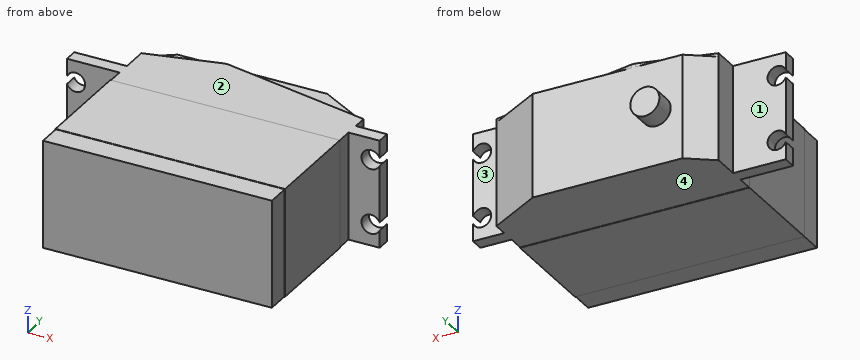
from build123d import *

# Parameters (mm, degrees)
SKETCH2_W            = 66
SKETCH2_H            = 31
BOSS_EXTRUDE1_DEPTH  = 44.6
SKETCH4_W            = 31
SKETCH4_H            = 3.9
BOSS_EXTRUDE2_DEPTH  = 9
SKETCH6_R            = 2.75
CUT_EXTRUDE3_DEPTH   = 64.193433203
BOSS_EXTRUDE4_DEPTH  = 3.9
SKETCH8_W            = 66
SKETCH8_H            = 31
BOSS_EXTRUDE5_DEPTH  = 12.96
CUT_EXTRUDE7_DEPTH   = 82.21610038
CUT_EXTRUDE8_DEPTH   = 82.21610038
CUT_EXTRUDE9_DEPTH   = 1
SKETCH12_R           = 4.19
BOSS_EXTRUDE6_DEPTH  = 6
SKETCH13_W           = 66
SKETCH13_H           = 29.265979079
BOSS_EXTRUDE7_DEPTH  = 0.1
SKETCH14_W           = 31.1
SKETCH14_H           = 29.164669929
BOSS_EXTRUDE8_DEPTH  = 0.1
SKETCH15_W           = 66.1
SKETCH15_H           = 29.164669929
BOSS_EXTRUDE9_DEPTH  = 0.1
SKETCH16_W           = 31.2
SKETCH16_H           = 29.265979079
BOSS_EXTRUDE10_DEPTH = 0.1


with BuildPart() as part:
    # Sketch2 → Boss-Extrude1 (new body)
    with BuildSketch(Plane(origin=(0, 0, 0), x_dir=(1, 0, 0), z_dir=(0, 1, 0))):
        Rectangle(SKETCH2_W, SKETCH2_H)
    extrude(amount=BOSS_EXTRUDE1_DEPTH)

    # Sketch4 → Boss-Extrude2 (add)
    with BuildSketch(Plane(origin=(33, 0, 0), x_dir=(0, 0, -1), z_dir=(1, 0, 0))):
        with Locations((0, 42.65)):
            Rectangle(SKETCH4_W, SKETCH4_H)
    extrude(amount=BOSS_EXTRUDE2_DEPTH)

    # Sketch6 → Cut-Extrude3 (cut, through all)
    with BuildSketch(Plane(origin=(0, 44.6, 0), x_dir=(1, 0, 0), z_dir=(0, 1, 0))):
        with Locations((39.5, -9.35)):
            Circle(SKETCH6_R)
        with Locations((39.5, 9.35)):
            Circle(SKETCH6_R)
    extrude(amount=-CUT_EXTRUDE3_DEPTH, mode=Mode.SUBTRACT)

    # Sketch7 → Boss-Extrude4 (add)
    with BuildSketch(Plane(origin=(0, 44.6, 0), x_dir=(1, 0, 0), z_dir=(0, 1, 0))):
        with BuildLine():
            Line((-33, 15.5), (-48.186111703, 15.5))
            Line((-48.186111703, 15.5), (-48.186111703, 10.495643924))
            ThreePointArc((-48.186111703, 10.495643924), (-42.936111703, 9.35), (-48.186111703, 8.204356076))
            Line((-48.186111703, 8.204356076), (-48.186111703, -8.204356076))
            ThreePointArc((-48.186111703, -8.204356076), (-42.936111703, -9.35), (-48.186111703, -10.495643924))
            Line((-48.186111703, -10.495643924), (-48.186111703, -15.5))
            Line((-48.186111703, -15.5), (-33, -15.5))
            Line((-33, -15.5), (-33, 15.5))
        make_face()
    extrude(amount=-BOSS_EXTRUDE4_DEPTH)

    # Sketch8 → Boss-Extrude5 (add)
    with BuildSketch(Plane(origin=(0, 44.6, 0), x_dir=(1, 0, 0), z_dir=(0, 1, 0))):
        Rectangle(SKETCH8_W, SKETCH8_H)
    extrude(amount=BOSS_EXTRUDE5_DEPTH)

    # Sketch9 → Cut-Extrude7 (cut, through all)
    with BuildSketch(Plane.XY.offset(15.5)):
        Polygon((-25.417976584, 57.56), (-33, 52.251010049), (-33, 57.56), align=None)
    extrude(amount=-CUT_EXTRUDE7_DEPTH, mode=Mode.SUBTRACT)

    # Sketch10 → Cut-Extrude8 (cut, through all)
    with BuildSketch(Plane.XY.offset(15.5)):
        Polygon((17.751890933, 57.56), (33, 48.756500125), (33, 57.56), align=None)
    extrude(amount=-CUT_EXTRUDE8_DEPTH, mode=Mode.SUBTRACT)

    # Sketch11 → Cut-Extrude9 (cut)
    with BuildSketch(Plane.XY.offset(15.5)):
        Polygon((-33, 52.251010049), (-11.889467425, 57.56), (-25.417976584, 57.56), align=None)
        Polygon((33, 48.756500125), (-10.755426907, 57.56), (17.751890933, 57.56), align=None)
    extrude(amount=-CUT_EXTRUDE9_DEPTH, mode=Mode.SUBTRACT)

    # Sketch12 → Boss-Extrude6 (add)
    with BuildSketch(Plane(origin=(0, 57.56, 0), x_dir=(1, 0, 0), z_dir=(0, 1, 0))):
        with Locations(Location((-17.839262747, 0, 0), (0, 0, 270))):
            Circle(SKETCH12_R)
    extrude(amount=BOSS_EXTRUDE6_DEPTH)

    # Sketch13 → Boss-Extrude7 (add)
    with BuildSketch(Plane(origin=(0, 0, -15.5), x_dir=(-1, 0, 0), z_dir=(0, 0, -1))):
        with Locations((0, 21.440452746)):
            Rectangle(SKETCH13_W, SKETCH13_H)
    extrude(amount=BOSS_EXTRUDE7_DEPTH)

    # Sketch14 → Boss-Extrude8 (add)
    with BuildSketch(Plane.ZY.offset(33)):
        with Locations((-0.05, 21.389798171)):
            Rectangle(SKETCH14_W, SKETCH14_H)
    extrude(amount=BOSS_EXTRUDE8_DEPTH)

    # Sketch15 → Boss-Extrude9 (add)
    with BuildSketch(Plane.XY.offset(15.5)):
        with Locations((-0.05, 21.389798171)):
            Rectangle(SKETCH15_W, SKETCH15_H)
    extrude(amount=BOSS_EXTRUDE9_DEPTH)

    # Sketch16 → Boss-Extrude10 (add)
    with BuildSketch(Plane(origin=(33, 0, 0), x_dir=(0, 0, -1), z_dir=(1, 0, 0))):
        with Locations((0, 21.440452746)):
            Rectangle(SKETCH16_W, SKETCH16_H)
    extrude(amount=BOSS_EXTRUDE10_DEPTH)


solid = part.part
Source: CAD feature listing. Evaluate the final solid. Frame: model axes, mm. Face numbers are marked on the shaded views. A direction names the side the tool comes from. Coordinates: 2 decimals unless noted, no trailing zeros. Loops run counter-clockwise (first coordinate to the right, second up) from the corner with the lowest first, then second, coordinate; pieces in that order, holes last. Notation, with made-up numbers: M 63.5,-27 L 94.5,-27 A33 cw 94.5,5 Z; hole C 24,-0.75 d10. An arc over 180 degrees is marked long. Answer in a Markdown table with one row per item.
Q1. Section D-D on y = 33. Return the cut outline in (x, z).
Answers below:
| item | result |
|---|---|
| outline | M -33.1,-15.6 L 33.1,-15.6 L 33.1,15.6 L -33.1,15.6 Z |
Q2. Set-up query: the marked faces 1, 2, 3 and 4. Return all of +Z, -Z, +X, -X, +Y, -Y with unobstructed straight access to the full face (end or side cutting, diameter ignored); none if empty.
Answers below:
| item | result |
|---|---|
| face 1 | +Z, -Z, -X, +Y |
| face 2 | +Z, +X, -X, +Y |
| face 3 | +Z, -Z, +X, +Y |
| face 4 | -Z, +X, -X, +Y |
Q3. Ray query, probe 1 along Y at (x, z) = (-11, 7); probe 2 along X at (y, z) = (11, -10); probe 3 along Z at (x, y) = (6.5, 5.5). Return the intervals inside material, ascending. Write a range as from..to.
Answers below:
| item | result |
|---|---|
| probe 1 | y = 0..57.56 |
| probe 2 | x = -33.1..33.1 |
| probe 3 | z = -15.5..15.5 |
Q4. Section B-B on z = -9.35. Return the cut outline in (x, y), plus the area to 3 significant figures.
Answers below:
| item | result |
|---|---|
| outline | M -42.94,40.7 L -33,40.7 L -33,35.97 L -33.1,35.97 L -33.1,6.81 L -33,6.81 L -33,0 L 33,0 L 33,6.81 L 33.1,6.81 L 33.1,36.07 L 33,36.07 L 33,40.7 L 36.75,40.7 L 36.75,44.6 L 33,44.6 L 33,48.76 L 17.75,57.56 L -25.42,57.56 L -33,52.25 L -33,44.6 L -42.94,44.6 Z |
| area | 3,770 mm^2 |
Q5. First-contact query: pin 1 (1 mm diameter, centred on y = 27, z = -4.5, fed in from +X); pin 2 (5.5 mm diameter, centred on x = 13.5, y = 3.5, fed in from -Z); pin 3 (10 mm diameter, centred on x = -25.5, z = 8, fed in from -Y); pin 4 (7.5 mm diameter, centred on y = 4, z = -5.5, fed in from -X). Flat tips, straight axial feed; report the tip coordinate or a pass-through.
Answers below:
| item | result |
|---|---|
| pin 1 | stops at x = 33.1 |
| pin 2 | stops at z = -15.5 |
| pin 3 | stops at y = 0 |
| pin 4 | stops at x = -33.1 |
Q6. Section C-C on z = 0. Return the cut outline in (x, y).
Answers below:
| item | result |
|---|---|
| outline | M -48.19,40.7 L -33,40.7 L -33,35.97 L -33.1,35.97 L -33.1,6.81 L -33,6.81 L -33,0 L 33,0 L 33,6.81 L 33.1,6.81 L 33.1,36.07 L 33,36.07 L 33,40.7 L 42,40.7 L 42,44.6 L 33,44.6 L 33,48.76 L 17.75,57.56 L -13.65,57.56 L -13.65,63.56 L -22.03,63.56 L -22.03,57.56 L -25.42,57.56 L -33,52.25 L -33,44.6 L -48.19,44.6 Z |
Q7. Section A-A on x = 39.5. Return the cut outline in (y, z).
Answers below:
| item | result |
|---|---|
| outline | M 40.7,-15.5 L 44.6,-15.5 L 44.6,-12.1 L 40.7,-12.1 Z; M 40.7,-6.6 L 44.6,-6.6 L 44.6,6.6 L 40.7,6.6 Z; M 40.7,12.1 L 44.6,12.1 L 44.6,15.5 L 40.7,15.5 Z |
